```python
from build123d import *

# Parameters (mm, degrees)
SKETCH1_W               = 17.9
SKETCH1_H               = 21.7
BOSS_EXTRUDE1_DEPTH     = 2
BOSS_EXTRUDE2_OUTLINE_W = 19.9
BOSS_EXTRUDE2_OUTLINE_H = 23.7
BOSS_EXTRUDE2_DEPTH     = 7
SKETCH3_W               = 10
SKETCH3_H               = 5
CUT_EXTRUDE1_DEPTH      = 1
SKETCH4_W               = 9.2
SKETCH4_H               = 5
CUT_EXTRUDE2_DEPTH      = 1
SKETCH7_W               = 5
SKETCH7_H               = 10
BOSS_EXTRUDE3_DEPTH     = 1.5
FILLET1_R               = 5
SKETCH8_W               = 4.35
SKETCH8_H               = 1.5
CUT_EXTRUDE4_DEPTH      = 1.7
FILLET3_R               = 2


# Read off the part's stored shape, not the designer's step: Boss-Extrude2
with BuildPart() as part:
    # Sketch1 → Boss-Extrude1 (new body)
    with BuildSketch(Plane(origin=(0, 0, 0), x_dir=(1, 0, 0), z_dir=(0, 1, 0))):
        Rectangle(SKETCH1_W, SKETCH1_H)
    extrude(amount=BOSS_EXTRUDE1_DEPTH)

    # Boss-Extrude2 outline → Boss-Extrude2 (add)
    with BuildSketch(Plane(origin=(0, 0, 0), x_dir=(1, 0, 0), z_dir=(0, 1, 0))):
        Rectangle(BOSS_EXTRUDE2_OUTLINE_W, BOSS_EXTRUDE2_OUTLINE_H)
        Polygon((4.6, -9.35), (4.6, -10.85), (-4.6, -10.85), (-4.6, -9.35), (-8.95, -9.35), (-8.95, 10.85), (8.95, 10.85), (8.95, -9.35), align=None, mode=Mode.SUBTRACT)
    extrude(amount=BOSS_EXTRUDE2_DEPTH)

    # Sketch3 → Cut-Extrude1 (cut)
    with BuildSketch(Plane.XY.offset(-10.85)):
        with Locations((0, 4.5)):
            Rectangle(SKETCH3_W, SKETCH3_H)
    extrude(amount=-CUT_EXTRUDE1_DEPTH, mode=Mode.SUBTRACT)

    # Sketch4 → Cut-Extrude2 (cut)
    with BuildSketch(Plane.XY.offset(11.85)):
        with Locations((0, 4.5)):
            Rectangle(SKETCH4_W, SKETCH4_H)
    extrude(amount=-CUT_EXTRUDE2_DEPTH, mode=Mode.SUBTRACT)

    # Sketch7 → Boss-Extrude3 (add)
    with BuildSketch(Plane(origin=(0, 7, 0), x_dir=(1, 0, 0), z_dir=(0, 1, 0))):
        with Locations((-12.45, 0)):
            Rectangle(SKETCH7_W, SKETCH7_H)
        with Locations((12.45, 0)):
            Rectangle(SKETCH7_W, SKETCH7_H)
    extrude(amount=-BOSS_EXTRUDE3_DEPTH)

    # Fillet1
    fillet1_edges = [part.edges().sort_by_distance(p)[0] for p in [
        (9.95, 5.5, 0),
        (-9.95, 5.5, 0),
    ]]
    fillet(fillet1_edges, radius=FILLET1_R - 0.0001)  # a hair under: the kernel refuses the full size

    # Sketch8 → Cut-Extrude4 (cut)
    with BuildSketch(Plane(origin=(0, 7, 0), x_dir=(1, 0, 0), z_dir=(0, 1, 0))):
        with Locations((-6.775, -10.1)):
            Rectangle(SKETCH8_W, SKETCH8_H)
        with Locations((6.775, -10.1)):
            Rectangle(SKETCH8_W, SKETCH8_H)
    extrude(amount=-CUT_EXTRUDE4_DEPTH, mode=Mode.SUBTRACT)

    # Fillet3
    fillet3_edges = [part.edges().sort_by_distance(p)[0] for p in [
        (-9.95, 3.5, 11.85),
        (9.95, 3.5, 11.85),
    ]]
    fillet(fillet3_edges, radius=FILLET3_R)


solid = part.part
```
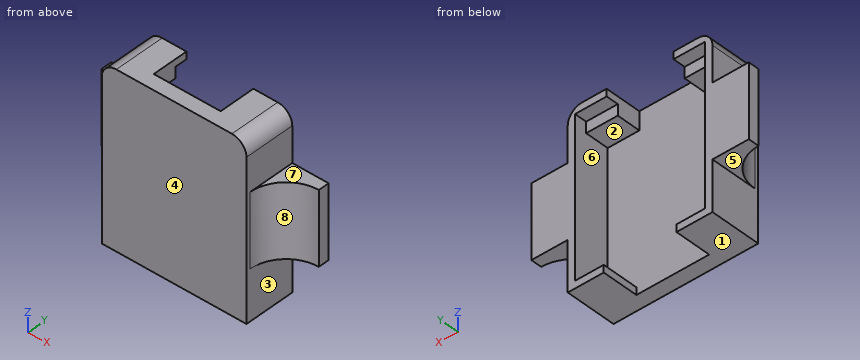
Could you check a few things on this model? Use its own coordinates, in mm. Face numbers are marked on the shaded views. A direction names the side the tool comes from. Coordinates: 2 decimals unless noted, no trailing zeros. Write each loop counter-clockwise with the first axis right and the second up, starting at its lowest first coordinate (ties: lowest second). Pieces come first, ordered by that corner, then holes. Notation, with made-up numbers: M 84,-1.75 L 140,-1.75 A34 cw 140,32.25 Z; hole C -28,-17.5 d9. An arc over 180 degrees is marked long. Answer as CSV lines item,"result". Start each with the question number.
1) I want a section at A-A, the plane y = 3.25. Please give me the cut outline in (x, z), and give its area (3 significant figures).
2) For the marked faces 4, 5, 6, 7 and 8, which set-ups out of +Z, -Z, +X, -X, +Y, -Y let a thin tool reach every point of the face, with its end or its side?
3) For P1, Ø1.5, axis at x = 12, y = 4, coming from the +Z side; P2, Ø0.5, axis at y = 3.5, z = -11.5, coming from the +X side; P3, Ø1.2, axis at x = -7, z = 10, coming from the +Y side, each with a flat end and sliding along its axis, tell me the tip position at first contact or that it passes through.
4) We'd pull the mould along X, two halves only. Please class the marked faces 1, 2 and 3: +X half, -X half, draft (parallel to the pull), parting line (faces both ways), or undercut.
5) I want a section at B-B, the plane x = -5.5. Please give me the cut outline in (y, z), and give its area (4 significant figures).
6) I want a section at C-C, the plane z = 7.5. Please give me the cut outline in (x, y), and give its area (3 significant figures).
7) Please list where these lines run through material, in increasing order: line 1 (Z direction, x = -7.25, y = 2.75); line 2 (X direction, y = 2.5, z = 5.75); line 3 (Y direction, x = 8.5, z = -5). Write a range as from..to.
Data:
1,outline,"M -10.77,-5 L -9.95,-5 L -9.95,-11.85 L -5,-11.85 L -5,-10.85 L -8.95,-10.85 L -8.95,9.35 L -4.6,9.35 L -4.6,11.85 L -7.95,11.85 A2 ccw -9.95,9.85 L -9.95,5 L -10.77,5 Z; M 4.6,9.35 L 8.95,9.35 L 8.95,-10.85 L 5,-10.85 L 5,-11.85 L 9.95,-11.85 L 9.95,-5 L 10.77,-5 L 10.77,5 L 9.95,5 L 9.95,9.85 A2 ccw 7.95,11.85 L 4.6,11.85 Z"
1,area,"91.8 mm^2"
2,face 4,"+Z, -Z, +X, -X, -Y"
2,face 5,"-Z, -X, +Y, -Y"
2,face 6,"+Y"
2,face 7,"+Z, +X, +Y, -Y"
2,face 8,"+Z, -Z, +X, -Y"
3,P1,"stops at z = 5"
3,P2,"stops at x = 9.95"
3,P3,"stops at y = 5.3"
4,face 1,"draft"
4,face 2,"undercut"
4,face 3,"+X half"
5,outline,"M 0,-11.85 L 7,-11.85 L 7,-10.85 L 2,-10.85 L 2,9.35 L 5.3,9.35 L 5.3,10.85 L 7,10.85 L 7,11.85 L 0,11.85 Z"
5,area,"62.35 mm^2"
6,outline,"M -9.95,0 L 9.95,0 L 9.95,7 L 8.95,7 L 8.95,2 L -8.95,2 L -8.95,7 L -9.95,7 Z"
6,area,"49.8 mm^2"
7,line 1,"z = -11.85..-10.85, 9.35..11.85"
7,line 2,"x = -9.95..-8.95, 8.95..9.95"
7,line 3,"y = 0..2"
